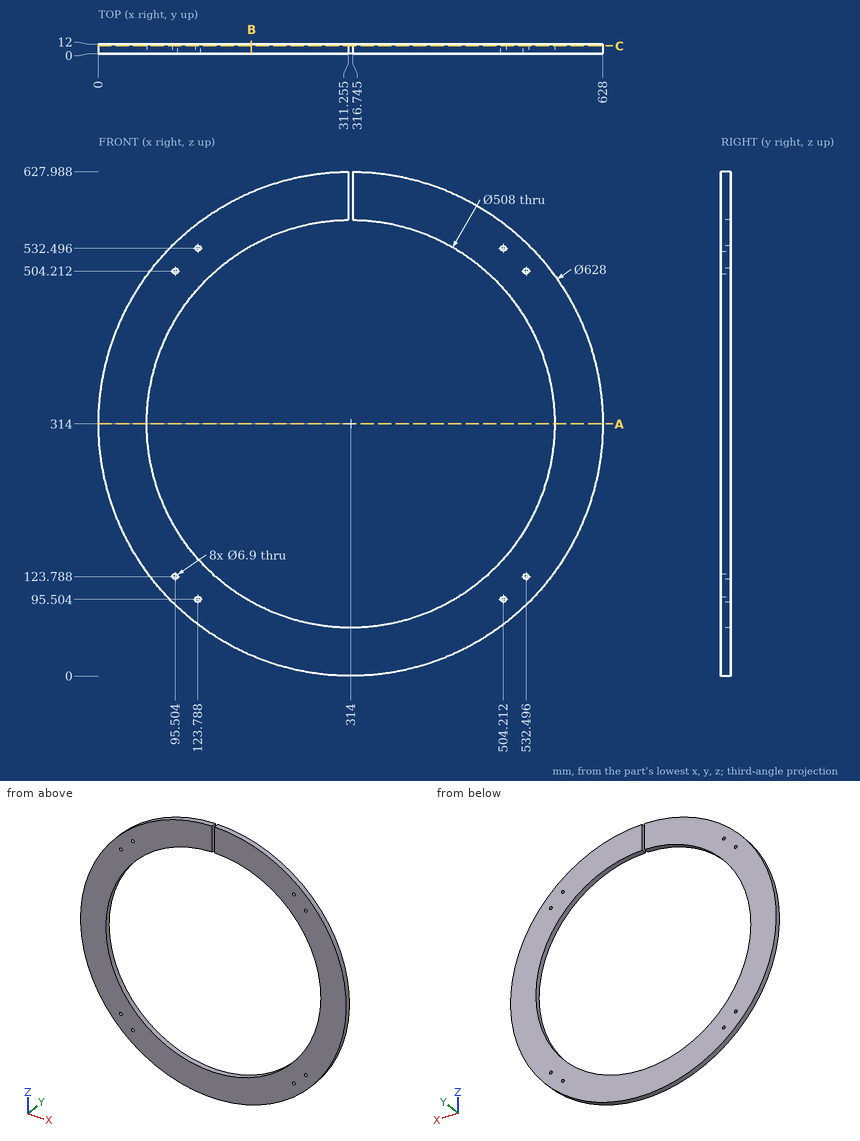
Geometry check sheet. Reference: drawing and pictorial views, mm from the part's lowest x, y, z. Coordinates: 2 decimals unless noted, no trailing zeros. Write each loop counter-clockwise with the first axis right and the second up, starting at its lowest first coordinate (ties: lowest second). Pieces come first, ordered by that corner, then holes.
Item 1: Scan lines: probe 1 along Z at (x, y) = (317, 11); probe 2 along Z at (x, y) = (229.5, 7.5); probe 3 along X at (y, z) = (4.75, 138.5) (1 decimal). Record each from-to range of solid material in increasing order.
Numbers:
probe 1: z = 0.01 to 60.02, 567.98 to 627.99
probe 2: z = 11.58 to 74.47, 553.53 to 616.42
probe 3: x = 53.6 to 130.4, 497.6 to 574.4
Item 2: Depth check by flat-ended pin: pin 1 Ø6 at (x, y) = (292, 5) entering from +Z; pin 2 Ø4 at (y, z) = (1.5, 481) entering from +X; pin 3 Ø5.5 at (x, z) = (95.5, 504.21) entering from +Y; pin 4 Ø6 at (y, z) = (8, 598.5) entering from +X. Enter the tip coordinate at first touch or a pass-through.
Numbers:
pin 1: stops at z = 627.42
pin 2: stops at x = 581.15
pin 3: passes through
pin 4: stops at x = 453.12
Item 3: Cross-section at C-C on y = 9.75. Count the separate pieces of the cut face and the enclosed holes in it, then the cut area to 3 significant figures.
Numbers:
separate pieces: 1
enclosed holes: 8
area: 106,000 mm2
Item 4: Cross-section at A-A on z = 314. Record the boundary of the cut face in (x, y).
Numbers:
outline: (0, 0) - (60, 0) - (60, 12) - (0, 12) - close; (568, 0) - (628, 0) - (628, 12) - (568, 12) - close
Item 5: Cross-section at B-B on x = 190.5. Record the boundary of the cut face in (y, z), then the cut area to 3 significant figures.
Numbers:
outline: (0, 25.31) - (12, 25.31) - (12, 92.05) - (0, 92.05) - close; (0, 535.95) - (12, 535.95) - (12, 602.69) - (0, 602.69) - close
area: 1,600 mm2
